The listing builds one solid part. Answer for the finished solid, in the listing's coordinates (mm). A direction names the side the tool comes from. Coordinates: 2 decimals unless noted, no trailing zeros. Order: outer loops, then holes, each group sorted by start corner. A loop starts at its lowest first (then second) coordinate and runs counter-clockwise, first axis right, second up. Notation, with made-up numbers: (46.25, 5.25) -> (53.25, 5.25) arc R23 ccw to (53.25, 21.25) -> close; hole circle Ø6 at (52, -14.75). An arc over 180 degrees is marked (long way). Return JSON: item names as keys, results as strings.
from build123d import *

# Parameters (mm, degrees)
F1_DEPTH = 8
F2_R     = 4.7625
F3_DEPTH = 19.05
F4_SIZE  = 1.27


with BuildPart() as f1:
    # F0 (on Front) → F1 (new body)
    with BuildSketch(Plane.XZ):
        Polygon((4.25, -7.361216), (8.5, 0), (4.25, 7.361216), (-4.25, 7.361216), (-8.5, 0), (-4.25, -7.361216), align=None)
    extrude(amount=F1_DEPTH)

    # F2 (on face) → F3 (join)
    with BuildSketch(Plane.XZ.offset(8)):
        Circle(F2_R)
    extrude(amount=F3_DEPTH)

    # F4
    f4_edges = [f1.edges().sort_by_distance(p)[0] for p in [
        (-4.7625, -27.05, 0),
        (6.375, 0, 3.680608),
        (0, 0, -7.361216),
        (6.375, 0, -3.680608),
        (-6.375, 0, -3.680608),
        (-6.375, 0, 3.680608),
        (0, 0, 7.361216),
        (6.375, -8, 3.680608),
        (6.375, -8, -3.680608),
        (4.7625, -17.525, 0),
        (-4.7625, -8, 0),
        (0, -8, 7.361216),
        (-6.375, -8, 3.680608),
        (0, -8, -7.361216),
        (-6.375, -8, -3.680608),
    ]]
    chamfer(f4_edges, length=F4_SIZE)


solid = f1.part
1. Each of these flat-tipped pins is pushed along its axis until it touches: pin 1 Ø5 at (x, y) = (0.5, -8) entering from +Z; pin 2 Ø1.5 at (y, z) = (-21.5, 1.5) entering from -X; pin 3 Ø2 at (y, z) = (-6.5, 4.5) entering from -X. Where does it stop, or does it pass through?
Answer block:
{"pin 1": "stops at z = 7.36", "pin 2": "stops at x = -4.7", "pin 3": "stops at x = -6.48"}
2. The part is cut by section A-A on x = 0. Give the vertices of the cut face in (y, z).
Answer block:
{"outline": "(-27.05, -3.49) -> (-25.78, -4.76) -> (-9.27, -4.76) -> (-8, -6.03) -> (-8, -6.09) -> (-6.73, -7.36) -> (-1.27, -7.36) -> (0, -6.09) -> (0, 6.09) -> (-1.27, 7.36) -> (-6.73, 7.36) -> (-8, 6.09) -> (-8, 6.03) -> (-9.27, 4.76) -> (-25.78, 4.76) -> (-27.05, 3.49) -> close"}
3. The part is cut by section C-C on z = 6.75. Give the vertices of the cut face in (x, y).
Answer block:
{"outline": "(-4.6, -6.73) -> (-3.9, -7.34) -> (3.9, -7.34) -> (4.6, -6.73) -> (4.6, -1.27) -> (3.9, -0.66) -> (-3.9, -0.66) -> (-4.6, -1.27) -> close"}
4. Consider line 1 (Y direction, x = -5.5, z = 2.5); line 2 (Z direction, x = 5.25, y = -1.25); line 3 (Y direction, x = -7.25, z = 1.25). Determine where each line is inside the solid, lowest interval first. Write a range as from..to.
Answer block:
{"line 1": "y = -8..0", "line 2": "z = -5.59..5.59", "line 3": "y = -7.19..-0.81"}
5. The part is cut by section B-B on y = -6. Give the vertices of the cut face in (x, z).
Answer block:
{"outline": "(-8.5, 0) -> (-4.25, -7.36) -> (4.25, -7.36) -> (8.5, 0) -> (4.25, 7.36) -> (-4.25, 7.36) -> close"}
6. The part is cut by section D-D on y = -18.75. Give the vertices of the cut face in (x, z) (1 decimal), and give its area (3 significant figures).
Answer block:
{"outline": "circle Ø9.5 at (0, 0)", "area": "71.3 mm2"}
7. For faces 1 (the face through (0.059, -7.356, 6.735)), 2 (the face through (-3.78, -17.41, -2.9)), determine the directions among +Z, -Z, +X, -X, +Y, -Y from which every point of the face is accessible in a straight line to the end or side of a thin tool.
Answer block:
{"face 1": "+Z, +X, -X, -Y", "face 2": "-Y"}
